Design review of the part built by this model. Coordinates are the model's own, in mm. Face numbers are marked on the shaded views. A direction names the side the tool comes from. Give positions to 0.01 mm unless a question says otherwise; leave off trailing zeros. Loops run counter-clockwise (first coordinate to the right, second up) from the corner with the lowest first, then second, coordinate; pieces in that order, holes last. Notation, with made-up numbers: M -16,4 L -1,4 A30 cw -1,32 Z; hole C -22,48.5 d11. An arc over 180 degrees is marked long. Use one line per item in the form item = value. Start each with the question number.
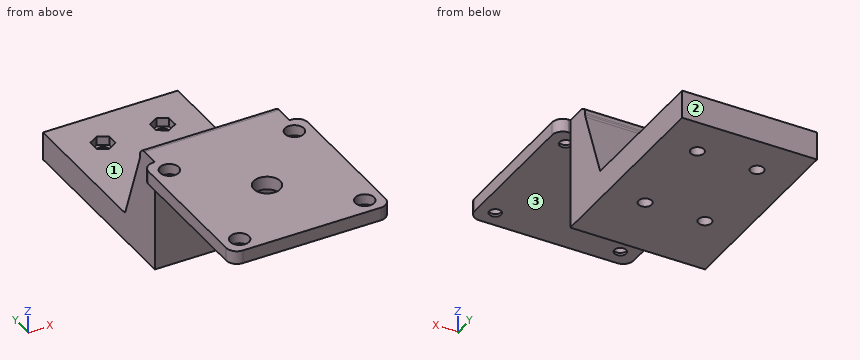
from build123d import *

# Parameters (mm, degrees)
SKETCH1_W           = 50.8
SKETCH1_H           = 65.000000038
SKETCH1_R           = 2.5
EXTRUDE_5_DEPTH     = 7.5
SKETCH1_3_W         = 50.8
SKETCH1_3_H         = 10
BOSS_EXTRUDE1_DEPTH = 34.125
BOSS_EXTRUDE2_START = 34.125
SKETCH1_4_R         = 2.25
BOSS_EXTRUDE2_DEPTH = 5
CHAMFER1_SIZE       = 10
CHAMFER1_SIZE2      = 27.474774195
FILLET1_R           = 3
SKETCH2_R           = 5
CUT_EXTRUDE1_DEPTH  = 144.721138443
SKETCH3_R           = 3.55
CUT_EXTRUDE2_DEPTH  = 4
CUT_EXTRUDE3_DEPTH  = 3.3
BOSS_EXTRUDE3_START = -3.18
SKETCH1_5_W         = 50.8
SKETCH1_5_H         = 65.000000038
SKETCH1_5_R         = 2.5
SKETCH1_5_H_2       = 10
BOSS_EXTRUDE3_DEPTH = 3.18


with BuildPart() as part:
    # Sketch1 → 5 (new body)
    with BuildSketch(Plane.XY):
        with Locations((0, 102.500000019)):
            Rectangle(SKETCH1_W, SKETCH1_H)
        with Locations((-11.25, 85.000000038)):
            Circle(SKETCH1_R, mode=Mode.SUBTRACT)
        with Locations((-11.25, 120.000000038)):
            Circle(SKETCH1_R, mode=Mode.SUBTRACT)
        with Locations((11.25, 85.000000038)):
            Circle(SKETCH1_R, mode=Mode.SUBTRACT)
        with Locations((11.25, 120.000000038)):
            Circle(SKETCH1_R, mode=Mode.SUBTRACT)
    extrude(amount=EXTRUDE_5_DEPTH)

    # Sketch1<3> → Boss-Extrude1 (add)
    with BuildSketch(Plane.XY):
        with Locations((0, 65)):
            Rectangle(SKETCH1_3_W, SKETCH1_3_H)
    extrude(amount=BOSS_EXTRUDE1_DEPTH)

    # Sketch1<4> → Boss-Extrude2 (add)
    with BuildSketch(Plane.XY.offset(BOSS_EXTRUDE2_START)):
        with BuildLine():
            Line((-25.4, 70), (-25.4, 60))
            Line((-25.4, 60), (-26, 60))
            ThreePointArc((-26, 60), (-28.828427125, 58.828427125), (-30, 56))
            Line((-30, 56), (-30, 4))
            ThreePointArc((-30, 4), (-28.828427125, 1.171572875), (-26, 0))
            Line((-26, 0), (26, 0))
            ThreePointArc((26, 0), (28.828427125, 1.171572875), (30, 4))
            Line((30, 4), (30, 56))
            ThreePointArc((30, 56), (28.828427125, 58.828427125), (26, 60))
            Line((26, 60), (25.4, 60))
            Line((25.4, 60), (25.4, 70))
            Line((25.4, 70), (-25.4, 70))
        make_face()
        with Locations((23.57, 53.57)):
            Circle(SKETCH1_4_R, mode=Mode.SUBTRACT)
        with Locations((-23.57, 6.43)):
            Circle(SKETCH1_4_R, mode=Mode.SUBTRACT)
        with Locations((-23.57, 53.57)):
            Circle(SKETCH1_4_R, mode=Mode.SUBTRACT)
        with Locations((23.57, 6.43)):
            Circle(SKETCH1_4_R, mode=Mode.SUBTRACT)
    extrude(amount=BOSS_EXTRUDE2_DEPTH)

    # Chamfer1
    chamfer1_edges = [part.edges().sort_by_distance(p)[0] for p in [
        (0, 70, 7.5),
    ]]
    chamfer1_side = [part.faces().sort_by_distance(p)[0] for p in [
        (0, 102.500000019, 7.5),
    ]]
    chamfer(chamfer1_edges, length=CHAMFER1_SIZE, length2=CHAMFER1_SIZE2, reference=chamfer1_side[0])

    # Fillet1
    fillet1_edges = [part.edges().sort_by_distance(p)[0] for p in [
        (0, 70, 39.125),
        (0, 70, 34.974774195),
    ]]
    fillet(fillet1_edges, radius=FILLET1_R)

    # Sketch2 → Cut-Extrude1 (cut, through all)
    with BuildSketch(Plane.XY.offset(39.125)):
        with Locations((0, 30)):
            Circle(SKETCH2_R)
    extrude(amount=-CUT_EXTRUDE1_DEPTH, mode=Mode.SUBTRACT)

    # Sketch3 → Cut-Extrude2 (cut)
    with BuildSketch(Plane.XY.offset(39.125)):
        with Locations((-23.57, 53.57)):
            Circle(SKETCH3_R)
        with Locations((23.57, 53.57)):
            Circle(SKETCH3_R)
        with Locations((-23.57, 6.43)):
            Circle(SKETCH3_R)
        with Locations((23.57, 6.43)):
            Circle(SKETCH3_R)
    extrude(amount=-CUT_EXTRUDE2_DEPTH, mode=Mode.SUBTRACT)

    # Sketch4 → Cut-Extrude3 (cut)
    with BuildSketch(Plane.XY.offset(7.5)):
        Polygon((-11.25, 124.156921976), (-14.85, 122.078461007), (-14.85, 117.921539069), (-11.25, 115.8430781), (-7.65, 117.921539069), (-7.65, 122.078461007), align=None)
        Polygon((11.25, 124.156921976), (7.65, 122.078461007), (7.65, 117.921539069), (11.25, 115.8430781), (14.85, 117.921539069), (14.85, 122.078461007), align=None)
        Polygon((-11.25, 89.156921976), (-14.85, 87.078461007), (-14.85, 82.921539069), (-11.25, 80.8430781), (-7.65, 82.921539069), (-7.65, 87.078461007), align=None)
        Polygon((11.25, 89.156921976), (7.65, 87.078461007), (7.65, 82.921539069), (11.25, 80.8430781), (14.85, 82.921539069), (14.85, 87.078461007), align=None)
    extrude(amount=-CUT_EXTRUDE3_DEPTH, mode=Mode.SUBTRACT)

    # Sketch1<5> → Boss-Extrude3 (add)
    # profile 1 of 2: a face of its own
    with BuildSketch(Plane.XY.offset(BOSS_EXTRUDE3_START)):
        with Locations((0, 102.500000019)):
            Rectangle(SKETCH1_5_W, SKETCH1_5_H)
        with Locations((-11.25, 85.000000038)):
            Circle(SKETCH1_5_R, mode=Mode.SUBTRACT)
        with Locations((-11.25, 120.000000038)):
            Circle(SKETCH1_5_R, mode=Mode.SUBTRACT)
        with Locations((11.25, 85.000000038)):
            Circle(SKETCH1_5_R, mode=Mode.SUBTRACT)
        with Locations((11.25, 120.000000038)):
            Circle(SKETCH1_5_R, mode=Mode.SUBTRACT)
    # profile 2 of 2: a face of its own
    with BuildSketch(Plane.XY.offset(BOSS_EXTRUDE3_START)):
        with Locations((0, 65)):
            Rectangle(SKETCH1_5_W, SKETCH1_5_H_2)
    extrude(amount=BOSS_EXTRUDE3_DEPTH)


solid = part.part
Q1. Take a section at B-B on y = 85. Give the boundary of the cut face in (x, z).
Q2. Clearance check with flat-ended pins moving along their axes: pin 1 Ø2 at (x, y) = (10, 87) entering from +Z; pin 2 Ø8 at (x, z) = (-13, 13.5) entering from +Y; pin 3 Ø3.5 at (y, z) = (84.5, 6.5) entering from -X. State where each tip first meets the part, or that it passes through.
Q3. Take a section at D-D on x = 16.5. Give the boundary of the cut face in (y, z) (3 decimals), plus the area to 3 significant figures.
Q4. For the marked faces 1, 2 and 3, list the 3-axis set-ups (+Z, -Z, +X, -X, +Y, -Y) from which the entire face can be reached by the end or side of a thin tool; tool diameter is ignored.
Q5. Wall thickness on probe 1 along Y at (x, z) = (-11.25, 1); probe 2 along Y at (x, z) = (-23.57, 37.05); probe 3 along Z at (x, y) = (-4, 114.5): over which ranges is each line inside the solid? List them lowest first.
Q6. Take a section at C-C on x = 0. Give the boundary of the cut face in (y, z) (3 decimals), plus the area to 3 significant figures.
Q7. Take a section at A-A on x = -23.57. Give the boundary of the cut face in (y, z) (3 decimals).
Response values:
q1.outline = M -25.4,-3.18 L -13.75,-3.18 L -13.75,4.2 L -14.85,4.2 L -14.85,7.5 L -25.4,7.5 Z; M -8.75,-3.18 L 8.75,-3.18 L 8.75,4.2 L 7.65,4.2 L 7.65,7.5 L -7.65,7.5 L -7.65,4.2 L -8.75,4.2 Z; M 13.75,-3.18 L 25.4,-3.18 L 25.4,7.5 L 14.85,7.5 L 14.85,4.2 L 13.75,4.2 Z
q2.pin_1 = 4.2
q2.pin_2 = 79.27
q2.pin_3 = -25.4
q3.outline = M 0,34.125 L 60,34.125 L 60,-3.18 L 135,-3.18 L 135,7.5 L 80,7.5 L 70.181,34.478 A3 cw 70,35.504 L 70,36.125 A3 ccw 67,39.125 L 0,39.125 Z
q3.area = 1,550 mm^2
q4.face_1 = +Z, +X, -X, +Y
q4.face_2 = +Z, -Z, +X, -X, +Y
q4.face_3 = -Z, +X, -X, -Y
q5.probe_1 = 60 to 82.5, 87.5 to 117.5, 122.5 to 135
q5.probe_2 = 0 to 2.88, 9.98 to 50.02, 57.12 to 69.85
q5.probe_3 = -3.18 to 7.5
q6.outline = M 0,34.125 L 25,34.125 L 25,39.125 L 0,39.125 Z; M 35,34.125 L 60,34.125 L 60,-3.18 L 135,-3.18 L 135,7.5 L 80,7.5 L 70.181,34.478 A3 cw 70,35.504 L 70,36.125 A3 ccw 67,39.125 L 35,39.125 Z
q6.area = 1,500 mm^2
q7.outline = M 0,34.125 L 4.18,34.125 L 4.18,35.125 L 2.88,35.125 L 2.88,39.125 L 0,39.125 Z; M 8.68,34.125 L 51.32,34.125 L 51.32,35.125 L 50.02,35.125 L 50.02,39.125 L 9.98,39.125 L 9.98,35.125 L 8.68,35.125 Z; M 55.82,34.125 L 60,34.125 L 60,-3.18 L 135,-3.18 L 135,7.5 L 80,7.5 L 70.181,34.478 A3 cw 70,35.504 L 70,36.125 A3 ccw 67,39.125 L 57.12,39.125 L 57.12,35.125 L 55.82,35.125 Z
